from build123d import *

# Parameters (mm, degrees)
SKETCH_1_W              = 36
SKETCH_1_H              = 18
EXTRUDE_1_DEPTH         = 8
CUT_EXTRUDE_1_DEPTH     = 38.960505792
CHAMFER_1_SIZE          = 2
CUT_EXTRUDE_2_DEPTH     = 22.656407828
CUT_EXTRUDE_START       = -2
CUT_EXTRUDE_3_OUTLINE_R = 2
CUT_EXTRUDE_3_DEPTH     = 2
EXTRUDE_2_DEPTH         = 0.2


# Read off the part's stored shape, not the designer's step: the extrude step
with BuildPart() as part:
    # Sketch 1 → Extrude 1 (new body)
    with BuildSketch(Plane(origin=(0, 0, 0), x_dir=(0, 0, -1), z_dir=(1, 0, 0))):
        Rectangle(SKETCH_1_W, SKETCH_1_H)
    extrude(amount=EXTRUDE_1_DEPTH)

    # Sketch 2 → Cut-Extrude 1 (cut, through all)
    with BuildSketch(Plane.XY.offset(18)):
        with BuildLine():
            ThreePointArc((0, -3.1), (3.1, 0), (0, 3.1))
            Line((0, 3.1), (0, -3.1))
        make_face()
    extrude(amount=-CUT_EXTRUDE_1_DEPTH, mode=Mode.SUBTRACT)

    # Chamfer 1
    chamfer_1_edges = [part.edges().sort_by_distance(p)[0] for p in [
        (8, 0, 18),
        (8, -9, 0),
        (8, 0, -18),
        (8, 9, 0),
    ]]
    chamfer(chamfer_1_edges, length=CHAMFER_1_SIZE)

    # Sketch 3 → Cut-Extrude 2 (cut, through all)
    with BuildSketch(Plane(origin=(8, 0, 0), x_dir=(0, 0, -1), z_dir=(1, 0, 0))):
        with BuildLine():
            ThreePointArc((1.413329403, 7), (1.552631161, 6.636440782), (1.6, 6.25))
            ThreePointArc((1.6, 6.25), (-0.386440782, 4.697368839), (-1.413329403, 7))
            Line((-1.413329403, 7), (-1.854049622, 7))
            ThreePointArc((-1.854049622, 7), (-0.382034525, 4.286826645), (2, 6.25))
            ThreePointArc((2, 6.25), (1.963173355, 6.632034525), (1.854049622, 7))
            Line((1.854049622, 7), (1.413329403, 7))
        make_face()
        with BuildLine():
            ThreePointArc((-1.413329403, 7), (0, 7.85), (1.413329403, 7))
            Line((1.413329403, 7), (1.854049622, 7))
            ThreePointArc((1.854049622, 7), (0, 8.25), (-1.854049622, 7))
            Line((-1.854049622, 7), (-1.413329403, 7))
        make_face()
        with BuildLine():
            ThreePointArc((-1.413329403, 7), (-0.386440782, 4.697368839), (1.6, 6.25))
            ThreePointArc((1.6, 6.25), (1.552631161, 6.636440782), (1.413329403, 7))
            Line((1.413329403, 7), (-1.413329403, 7))
        make_face()
        with BuildLine():
            Line((-1.413329403, 7), (1.413329403, 7))
            ThreePointArc((1.413329403, 7), (0, 7.85), (-1.413329403, 7))
        make_face()
        with BuildLine():
            ThreePointArc((-1.413329403, -7), (-0.386440782, -4.697368839), (1.6, -6.25))
            ThreePointArc((1.6, -6.25), (1.552631161, -6.636440782), (1.413329403, -7))
            Line((1.413329403, -7), (1.854049622, -7))
            ThreePointArc((1.854049622, -7), (1.963173355, -6.632034525), (2, -6.25))
            ThreePointArc((2, -6.25), (-0.382034525, -4.286826645), (-1.854049622, -7))
            Line((-1.854049622, -7), (-1.413329403, -7))
        make_face()
        with BuildLine():
            ThreePointArc((1.413329403, -7), (0, -7.85), (-1.413329403, -7))
            Line((-1.413329403, -7), (-1.854049622, -7))
            ThreePointArc((-1.854049622, -7), (0, -8.25), (1.854049622, -7))
            Line((1.854049622, -7), (1.413329403, -7))
        make_face()
        with BuildLine():
            ThreePointArc((1.413329403, -7), (1.552631161, -6.636440782), (1.6, -6.25))
            ThreePointArc((1.6, -6.25), (-0.386440782, -4.697368839), (-1.413329403, -7))
            Line((-1.413329403, -7), (1.413329403, -7))
        make_face()
        with BuildLine():
            Line((1.413329403, -7), (-1.413329403, -7))
            ThreePointArc((-1.413329403, -7), (0, -7.85), (1.413329403, -7))
        make_face()
    extrude(amount=-CUT_EXTRUDE_2_DEPTH, mode=Mode.SUBTRACT)

    # Cut-Extrude 3 outline → Cut-Extrude 3 (cut)
    # profile 1 of 2: a face of its own
    with BuildSketch(Plane(origin=(8, 0, 0), x_dir=(0, 0, -1), z_dir=(1, 0, 0)).offset(CUT_EXTRUDE_START)):
        with BuildLine():
            Line((-3, 9), (-3, 6.25))
            ThreePointArc((-3, 6.25), (0, 3.25), (3, 6.25))
            Line((3, 6.25), (3, 9))
            Line((3, 9), (-3, 9))
        make_face()
        with Locations((0, 6.25)):
            Circle(CUT_EXTRUDE_3_OUTLINE_R, mode=Mode.SUBTRACT)
    # profile 2 of 2: a face of its own
    with BuildSketch(Plane(origin=(8, 0, 0), x_dir=(0, 0, -1), z_dir=(1, 0, 0)).offset(CUT_EXTRUDE_START)):
        with BuildLine():
            Line((3, -9), (3, -6.25))
            ThreePointArc((3, -6.25), (0, -3.25), (-3, -6.25))
            Line((-3, -6.25), (-3, -9))
            Line((-3, -9), (3, -9))
        make_face()
        with Locations((0, -6.25)):
            Circle(CUT_EXTRUDE_3_OUTLINE_R, mode=Mode.SUBTRACT)
    extrude(amount=CUT_EXTRUDE_3_DEPTH, mode=Mode.SUBTRACT)

    # Sketch 5 → Extrude 2 (add)
    with BuildSketch(Plane(origin=(6, 0, 0), x_dir=(0, 0, -1), z_dir=(1, 0, 0))):
        with BuildLine():
            Line((3, 9), (-3, 9))
            Line((-3, 9), (-3, 6.25))
            ThreePointArc((-3, 6.25), (0, 3.25), (3, 6.25))
            Line((3, 6.25), (3, 9))
        make_face()
        with BuildLine():
            Line((-3, -9), (3, -9))
            Line((3, -9), (3, -6.25))
            ThreePointArc((3, -6.25), (0, -3.25), (-3, -6.25))
            Line((-3, -6.25), (-3, -9))
        make_face()
    extrude(amount=EXTRUDE_2_DEPTH)


solid = part.part
CAD build for the part. Positions are in the model's coordinates, mm. A direction names the side the tool comes from. Round coordinates to 2 decimals unless told otherwise and drop trailing zeros. Write each loop counter-clockwise with the first axis right and the second up, starting at its lowest first coordinate (ties: lowest second). Pieces come first, ordered by that corner, then holes. Notation, with made-up numbers: M 60.25,-21.5 L 110.25,-21.5 A22 cw 110.25,-12.5 Z; hole C 44,74 d8. An arc over 180 degrees is marked long. Put each result on its own line as item: value. Start each with the question number.
1) Drill centre lines: probe 1 along Z at (x, y) = (2.2, -6.25); probe 2 along X at (y, z) = (-3.75, -1); probe 3 along Y at (x, z) = (2, -12.5). Where is each one in solid material? Low to high. Write a range as [from, to].
2) Saw through at A-A, the plane x = 2.5. Write the cut outline in (y, z), and give its area (3 significant figures).
3) Saw through at B-B, the plane z = 0. Write the cut outline in (x, y), and give its area (3 significant figures).
4) Saw through at C-C, the plane y = 0. Write the cut outline in (x, z), and give its area (3 significant figures).
5) Saw through at D-D, the plane x = 1. Write the cut outline in (y, z).
6) 3-axis set-ups, long thin cutter, end or side, ignore diameter. For faces 4 (the cylindrical face through (7.09, 3.25, 0.07)), 5 (the flat face through (7, -7, -3)), 6 (the flat face through (6, 6, 0)), 7 (the flat face through (7, -8, 11)): which of +Z, -Z, +X, -X, +Y, -Y reach the whole face in a straight line?
7) Pull direction Y, two halves, no side cores. Call faces 1 (the flat face through (6, -6, 0)), 2 (the flat face through (0, -4, 0)), 3 (the flat face through (7, 8, 11)): pulls with the +Y half, pulls with the -Y half, needs draft (parallel to the pull), parting line crosses it, or undercut.
8) Pin check, flat tips, straight feed: pin 1 Ø3 at (y, z) = (5.5, 1) entering from +X; pin 2 Ø0.9 at (x, y) = (7, -7.5) entering from -Z; pin 3 Ø1.2 at (y, z) = (-5.5, 1) entering from -X. Stop position of each tip, or through.
Resolved:
1. probe 1: [-18, -2], [2, 18]
1. probe 2: [0, 6.2]
1. probe 3: [-9, -2.37], [2.37, 9]
2. outline: M -9,-18 L -1.83,-18 L -1.83,18 L -9,18 Z; M 1.83,-18 L 9,-18 L 9,18 L 1.83,18 Z; hole C -6.25,0 d4; hole C 6.25,0 d4
2. area: 491 mm²
3. outline: M 0,-9 L 6.2,-9 L 6.2,-3.25 L 8,-3.25 L 8,3.25 L 6.2,3.25 L 6.2,9 L 0,9 L 0,8.25 L 6,8.25 L 6,4.25 L 0,4.25 L 0,3.1 A3.1 cw 0,-3.1 L 0,-4.25 L 6,-4.25 L 6,-8.25 L 0,-8.25 Z
3. area: 60.2 mm²
4. outline: M 3.1,-18 L 6,-18 L 8,-16 L 8,16 L 6,18 L 3.1,18 Z
4. area: 172 mm²
5. outline: M -9,-18 L -2.93,-18 L -2.93,18 L -9,18 Z; M 2.93,-18 L 9,-18 L 9,18 L 2.93,18 Z; hole C -6.25,0 d4; hole C 6.25,0 d4
6. face 4: +X, +Y
6. face 5: +X, -Y
6. face 6: -X
6. face 7: +Z, +X, -Y
7. face 1: undercut
7. face 2: needs draft
7. face 3: pulls with the +Y half
8. pin 1: x = 6.2
8. pin 2: z = -17.45
8. pin 3: x = 6
